from build123d import *

# Parameters (mm, degrees)
F1_DEPTH      = 2
F2_DEPTH      = 2
F2_DEPTH_BACK = 3
F3_R          = 1.5
F4_R          = 1


with BuildPart() as f1:
    # F0 (on Top) → F1 (new body)
    with BuildSketch(Plane.XY):
        with BuildLine():
            ThreePointArc((15.0004277623, -9.0131663109), (16.8635329312, -4.6766715814), (17.5, 0))
            ThreePointArc((17.5, 0), (16.8635329312, 4.6766715814), (15.0004277623, 9.0131663109))
            ThreePointArc((15.0004277623, 9.0131663109), (14.1577974016, 10.2862419151), (13.2074176539, 11.4810330073))
            ThreePointArc((13.2074176539, 11.4810330073), (5.4077974016, 16.6434890352), (-3.936643451, 17.0514761337))
            ThreePointArc((-3.936643451, 17.0514761337), (-5.4077974016, 16.6434890352), (-6.8377947486, 16.1088349354))
            ThreePointArc((-6.8377947486, 16.1088349354), (-14.1577974016, 10.2862419151), (-17.4334072166, 1.5252254981))
            ThreePointArc((-17.4334072166, 1.5252254981), (-17.5, 0), (-17.4334072166, -1.5252254981))
            ThreePointArc((-17.4334072166, -1.5252254981), (-14.1577974016, -10.2862419151), (-6.8377947486, -16.1088349354))
            ThreePointArc((-6.8377947486, -16.1088349354), (-5.4077974016, -16.6434890352), (-3.936643451, -17.0514761337))
            ThreePointArc((-3.936643451, -17.0514761337), (5.4077974016, -16.6434890352), (13.2074176539, -11.4810330073))
            ThreePointArc((13.2074176539, -11.4810330073), (14.1577974016, -10.2862419151), (15.0004277623, -9.0131663109))
        make_face()
    extrude(amount=F1_DEPTH)

    # F0 (on Top) → F2 (join, two sides)
    with BuildSketch(Plane.XY) as f2_sk:
        with BuildLine():
            ThreePointArc((15.0004277623, 9.0131663109), (16.8635329312, 4.6766715814), (17.5, 0))
            ThreePointArc((17.5, 0), (16.8635329312, -4.6766715814), (15.0004277623, -9.0131663109))
            Line((15.0004277623, -9.0131663109), (17.143346014, -10.3007614982))
            ThreePointArc((17.143346014, -10.3007614982), (20, 0), (17.143346014, 10.3007614982))
            Line((17.143346014, 10.3007614982), (15.0004277623, 9.0131663109))
        make_face()
        with BuildLine():
            ThreePointArc((-3.936643451, 17.0514761337), (5.4077974016, 16.6434890352), (13.2074176539, 11.4810330073))
            Line((13.2074176539, 11.4810330073), (15.0941916045, 13.1211805798))
            ThreePointArc((15.0941916045, 13.1211805798), (6.1803398875, 19.0211303259), (-4.4990210869, 19.4874012957))
            Line((-4.4990210869, 19.4874012957), (-3.936643451, 17.0514761337))
        make_face()
        with BuildLine():
            ThreePointArc((-17.4334072166, 1.5252254981), (-14.1577974016, 10.2862419151), (-6.8377947486, 16.1088349354))
            Line((-6.8377947486, 16.1088349354), (-7.8146225698, 18.410097069))
            ThreePointArc((-7.8146225698, 18.410097069), (-16.1803398875, 11.7557050458), (-19.9238939618, 1.743114855))
            Line((-19.9238939618, 1.743114855), (-17.4334072166, 1.5252254981))
        make_face()
        with BuildLine():
            Line((-7.8146225698, -18.410097069), (-6.8377947486, -16.1088349354))
            ThreePointArc((-6.8377947486, -16.1088349354), (-14.1577974016, -10.2862419151), (-17.4334072166, -1.5252254981))
            Line((-17.4334072166, -1.5252254981), (-19.9238939618, -1.743114855))
            ThreePointArc((-19.9238939618, -1.743114855), (-16.1803398875, -11.7557050458), (-7.8146225698, -18.410097069))
        make_face()
        with BuildLine():
            Line((15.0941916045, -13.1211805798), (13.2074176539, -11.4810330073))
            ThreePointArc((13.2074176539, -11.4810330073), (5.4077974016, -16.6434890352), (-3.936643451, -17.0514761337))
            Line((-3.936643451, -17.0514761337), (-4.4990210869, -19.4874012957))
            ThreePointArc((-4.4990210869, -19.4874012957), (6.1803398875, -19.0211303259), (15.0941916045, -13.1211805798))
        make_face()
    extrude(amount=F2_DEPTH)
    extrude(f2_sk.sketch, amount=-F2_DEPTH_BACK)

    # F3
    f3_edges = [f1.edges().sort_by_distance(p)[0] for p in [
        (-17.433407, 1.525225, 1),
        (-17.433407, -1.525225, 1),
        (-3.936643, -17.051476, 1),
        (-6.837795, -16.108835, 1),
        (15.000428, -9.013166, 1),
        (13.207418, -11.481033, 1),
        (13.207418, 11.481033, 1),
        (15.000428, 9.013166, 1),
        (-6.837795, 16.108835, 1),
        (-3.936643, 17.051476, 1),
    ]]
    fillet(f3_edges, radius=F3_R)

    # F4
    f4_edges = [f1.edges().sort_by_distance(p)[0] for p in [
        (15.094192, -13.121181, -0.5),
        (17.143346, -10.300761, -0.5),
        (17.143346, 10.300761, -0.5),
        (15.094192, 13.121181, -0.5),
        (-4.499021, 19.487401, -0.5),
        (-7.814623, 18.410097, -0.5),
        (-19.923894, 1.743115, -0.5),
        (-19.923894, -1.743115, -0.5),
        (-4.499021, -19.487401, -0.5),
        (-7.814623, -18.410097, -0.5),
    ]]
    fillet(f4_edges, radius=F4_R)


solid = f1.part
Here's how the part is built. I have some questions about the finished solid (model axes, mm). A direction names the side the tool comes from. Round coordinates to 2 decimals unless told otherwise and drop trailing zeros. Write each loop counter-clockwise with the first axis right and the second up, starting at its lowest first coordinate (ties: lowest second). Pieces come first, ordered by that corner, then holes.
1. If we mould it in two halves opening along X, with no side actions, what happens to faces 6 (the cylindrical face through (17.057, 9.875, -0.535)), 7 (the flat face through (-14.3, 10.5, -3)), 8 (the cylindrical face through (14.662, -13.148, -0.535))? For each: released by +X, released by -X, zero draft, split by the parting line, or undercut.
2. Will these pins go through, and if not, where does the flat tip stop? pin 1 Ø3 at (x, z) = (12.5, -1.5) entering from +Y; pin 2 Ø2 at (y, z) = (15, 0) entering from -X; pin 3 Ø2 at (x, y) = (6, -15) entering from -Z.
3. Suppose I cut it at C-C (y = 5). List the corners of the cut face in (x, z) for me, and give its area (3 significant figures).
4. Suppose I cut it at B-B (x = -3). List the corners of the cut face in (y, z) for me.
5. For faces 1 (the cylindrical face through (-4.41, -17.39, 1.01)), 2 (the cylindrical face through (5.534, -16.602, -1.479)), 3 (the cylindrical face through (-7.973, 18.007, -0.465)), 4 (the flat face through (13.77, -11.97, -1.65)), 5 (the flat face through (-7.122, 16.778, -1.576)), which set-ups out of +Z, -Z, +X, -X, +Y, -Y let a thin tool reach every point of the face, with its end or its side?
6. I need wall thicknesses on L1, parallel to Y at x = 0, z = -2.25; L2, parallel to Z at x = -15, y = -4; L3, parallel to X at y = -9, z = -1.9. Which ranges of each line are inside material? Lowest first, please.
7. Suppose I cut it at A-A (z = -0.55). State how many separate pieces and enclosed holes the cut face has, and give its area (3 significant figures).
Answer sheet:
1. face 6: undercut
1. face 7: zero draft
1. face 8: released by +X
2. pin 1: stops at y = 16.7
2. pin 2: stops at x = -14.28
2. pin 3: stops at z = 0
3. outline: (-19.36, -3) - (-16.77, -3) - (-16.77, 0) - (16.77, 0) - (16.77, -3) - (19.36, -3) - (19.36, 2) - (-19.36, 2) - close
3. area: 93.0 mm2
4. outline: (-19.77, -3) - (-17.24, -3) - (-17.24, 0) - (17.24, 0) - (17.24, -3) - (19.77, -3) - (19.77, 2) - (-19.77, 2) - close
5. face 1: +Z, -Z
5. face 2: -Z
5. face 3: +Z, -Z, +Y
5. face 4: -Z, +X
5. face 5: -Z, +Y
6. L1: y = -20 to -17.5, 17.5 to 20
6. L2: z = 0 to 2
6. L3: x = -17.86 to -15.01, 15.01 to 17.86
7. separate pieces: 5
7. enclosed holes: 0
7. area: 251 mm2
